Autodesk Inventor part; units mm, degrees
sketch "スケッチ1" plane through (0, 0, 0) normal (0, 0, 1) x (1, 0, 0)
  circle A0 centre (0, 0) radius 10
  line L0 (-23.5, 23.5) -> (23.5, 23.5)
  line L1 (23.5, 23.5) -> (23.5, -23.5)
  line L2 (23.5, -23.5) -> (-23.5, -23.5)
  line L3 (-23.5, -23.5) -> (-23.5, 23.5)
  line L4 (-23.5, 23.5) -> (23.5, -23.5) construction
  line L5 (23.5, 23.5) -> (-23.5, -23.5) construction
  dimension "d0" = 20
  dimension "d1" = 47
  dimension "d2" = 47
extrude "押し出し1" add sketch "スケッチ1" along normal blind 13
properties part number "bearing1b"
Verification items for the finished model (mm, model axes). Give positions to 0.01 mm unless a question says otherwise; leave off trailing zeros. Order: outer loops, then holes, each group sorted by start corner. A loop starts at its lowest first (then second) coordinate and runs counter-clockwise, first axis right, second up. Notation, with made-up numbers: (51.5, 51) -> (93.5, 51) arc R12 cw to (93.5, 58) -> close; hole circle Ø3 at (25.25, 10). An arc over 180 degrees is marked (long way). Use a Markdown table: item, result.
1) Section check A-A, the plane y = 0. Record the boundary of the cut face in (x, z).
Results:
| item | result |
|---|---|
| outline | (-23.5, 0) -> (-10, 0) -> (-10, 13) -> (-23.5, 13) -> close; (10, 0) -> (23.5, 0) -> (23.5, 13) -> (10, 13) -> close |
2) Section check C-C, the plane z = 2.5. Record the boundary of the cut face in (x, y).
Results:
| item | result |
|---|---|
| outline | (-23.5, -23.5) -> (23.5, -23.5) -> (23.5, 23.5) -> (-23.5, 23.5) -> close; hole circle Ø20 at (0, 0) |
3) Material ranges on probe 1 along Y at (x, z) = (0, 3); probe 2 along Y at (x, z) = (8, 11.75); probe 3 along X at (y, z) = (4.5, 12.25), recorded low to high.
Results:
| item | result |
|---|---|
| probe 1 | -23.5 to -10, 10 to 23.5 |
| probe 2 | -23.5 to -6, 6 to 23.5 |
| probe 3 | -23.5 to -8.93, 8.93 to 23.5 |
